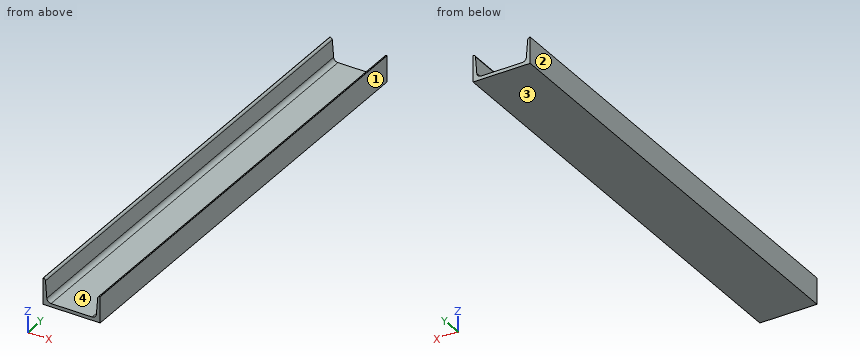
```python
from build123d import *

# Parameters (mm, degrees)
F1_DEPTH = 965


with BuildPart() as f1:
    # F0 (on Front) → F1 (new body)
    with BuildSketch(Plane.XZ):
        with BuildLine():
            Line((0.645623, 55), (0, 55))
            Line((0, 55), (0, 0))
            Line((0, 0), (120, 0))
            Line((120, 0), (120, 55))
            Line((120, 55), (119.354377, 55))
            ThreePointArc((119.354377, 55), (116.301906, 53.806421), (114.868708, 50.858854))
            Line((114.868708, 50.858854), (112.022583, 15.282293))
            ThreePointArc((112.022583, 15.282293), (109.156188, 9.387158), (103.051246, 7))
            Line((103.051246, 7), (16.948754, 7))
            ThreePointArc((16.948754, 7), (10.843812, 9.387158), (7.977417, 15.282293))
            Line((7.977417, 15.282293), (5.131292, 50.858854))
            ThreePointArc((5.131292, 50.858854), (3.698094, 53.806421), (0.645623, 55))
        make_face()
    extrude(amount=F1_DEPTH)


solid = f1.part
```
Here's how the part is built. I have some questions about the finished solid (model axes, mm). Face numbers are marked on the shaded views. Round coordinates to 2 decimals unless told otherwise and drop trailing zeros. Loops run counter-clockwise (first coordinate to the right, second up) from the corner with the lowest first, then second, coordinate; pieces in that order, holes last.
1. Suppose I cut it at A-A, the plane z = 26.5. Please give me the cut outline in (x, y).
Answers:
outline: (0, -965) - (7.08, -965) - (7.08, 0) - (0, 0) - close; (112.92, -965) - (120, -965) - (120, 0) - (112.92, 0) - close
2. Suppose I cut it at B-B, the plane y = -463.5. Please give me the cut outline in (x, z), and give its area (3 significant figures).
Answers:
outline: (0, 0) - (120, 0) - (120, 55) - (119.35, 55) arc R4.5 ccw to (114.87, 50.86) - (112.02, 15.28) arc R9 cw to (103.05, 7) - (16.95, 7) arc R9 cw to (7.98, 15.28) - (5.13, 50.86) arc R4.5 ccw to (0.65, 55) - (0, 55) - close
area: 1,510 mm2
3. Will these pins go through, and if not, where does the flat tip stop? pin 1 (12 mm diameter, centred on x = 21, y = -178.5, fed in from +Z); pin 2 (10 mm diameter, centred on x = 89.5, y = -566.5, fed in from +Z).
Answers:
pin 1: stops at z = 7.21
pin 2: stops at z = 7
4. If I drill on probe 1 along X at (y, z) = (-251.5, 14.5); probe 2 along Z at (x, y) = (58, -653); probe 3 along X at (y, z) = (-189, 21.5), over which ranges is the centre line in solid material (lowest first)?
Answers:
probe 1: x = 0 to 8.07, 111.93 to 120
probe 2: z = 0 to 7
probe 3: x = 0 to 7.48, 112.52 to 120
5. Suppose I cut it at C-C, the plane x = 56.5. Please give me the cut outline in (y, z).
Answers:
outline: (-965, 0) - (0, 0) - (0, 7) - (-965, 7) - close
6. Thinking about a two-plate mould opening in X: for the marked faces 1, 2, 3 and 4, which applies, released by +X, released by -X, zero draft, split by the parting line, or undercut?
Answers:
face 1: released by +X
face 2: released by -X
face 3: zero draft
face 4: undercut
